Part model, mm, in its own coordinate system. A direction names the side the tool comes from. Round coordinates to 2 decimals unless told otherwise and drop trailing zeros. Loops run counter-clockwise (first coordinate to the right, second up) from the corner with the lowest first, then second, coordinate; pieces in that order, holes last. Notation, with made-up numbers: (54.25, -21.75) - (76.25, -21.75) arc R16 ccw to (76.25, -10.75) - close; hole circle Ø11 at (-29.5, 23.25). An arc over 180 degrees is marked (long way). Write each question's results on one line, items separated by ' | '. Start each with the question number.
(1) Cut at A-A, the plane z = 3.5. List the corners of the cut face in (x, y), then the cut area to 3 significant figures.
(2) Drill centre lines: L1, parallel to Y at x = -1.5, z = 21.5; L2, parallel to X at y = 9, z = 14.75; L3, parallel to X at y = 0, z = 23.15. Where is each one in solid material? Low to high.
(3) Tool access for faces 1 (the face through (8.64, -10.69, 23.73)), 2 (the face through (-1, 18.911, 11)): list every direction of +Z, -Z, +X, -X, +Y, -Y with a clear straight run to the whole face (end or side of a thin tool).
(4) Cut at B-B, the plane y = -11. List the corners of the cut face in (x, z).
(5) Cut at D-D, the plane y = -16. List the corners of the cut face in (x, z), then the cut area to 3 significant figures.
(6) Mould opens along Y. For faces 3 (the face through (-1, -18.911, 11)), 4 (the face through (-11, 5, 25)), 5 (the face through (-1, 21.411, 12)), 6 (the face through (-43.589, 0, 11)) say: released by +Y, released by -Y, zero draft, split by the parting line, or undercut.
(7) Cut at C-C, the plane x = 8. List the corners of the cut face in (y, z), then the cut area to 3 significant figures.
from build123d import *

# Parameters (mm, degrees)
F0_W     = 92.177428
F0_H     = 42.82258
F1_DEPTH = 25
F2_T     = -2.5
F3_R     = 12.678487
F4_DEPTH = 73.8


with BuildPart() as f1:
    # F0 (on Top) → F1 (new body)
    with BuildSketch(Plane.XY):
        Rectangle(F0_W, F0_H)
    extrude(amount=F1_DEPTH)

    # F2
    f2_openings = [f1.faces().sort_by_distance(p)[0] for p in [
        (0, 0, 0),
    ]]
    offset(amount=F2_T, openings=f2_openings)

    # F3 (on face) → F4 (cut)
    with BuildSketch(Plane(origin=(0, 0, 22.5), x_dir=(1, 0, 0), z_dir=(0, 0, -1))):
        with Locations((1.825314, 0)):
            Circle(F3_R)
    extrude(amount=-F4_DEPTH, mode=Mode.SUBTRACT)


solid = f1.part
A:
1) outline: (-46.09, -21.41) - (46.09, -21.41) - (46.09, 21.41) - (-46.09, 21.41) - close; hole (-43.59, -18.91) - (43.59, -18.91) - (43.59, 18.91) - (-43.59, 18.91) - close | area: 650 mm2
2) L1: -21.41 to -18.91, 18.91 to 21.41 | L2: -46.09 to -43.59, 43.59 to 46.09 | L3: -46.09 to -10.85, 14.5 to 46.09
3) face 1: +Z, -Z | face 2: -Z
4) outline: (-46.09, 0) - (-43.59, 0) - (-43.59, 22.5) - (-4.48, 22.5) - (-4.48, 25) - (-46.09, 25) - close; (8.13, 22.5) - (43.59, 22.5) - (43.59, 0) - (46.09, 0) - (46.09, 25) - (8.13, 25) - close
5) outline: (-46.09, 0) - (-43.59, 0) - (-43.59, 22.5) - (43.59, 22.5) - (43.59, 0) - (46.09, 0) - (46.09, 25) - (-46.09, 25) - close | area: 343 mm2
6) face 3: undercut | face 4: zero draft | face 5: released by +Y | face 6: undercut
7) outline: (-21.41, 0) - (-18.91, 0) - (-18.91, 22.5) - (-11.07, 22.5) - (-11.07, 25) - (-21.41, 25) - close; (11.07, 22.5) - (18.91, 22.5) - (18.91, 0) - (21.41, 0) - (21.41, 25) - (11.07, 25) - close | area: 164 mm2
